from build123d import *

# Parameters (mm, degrees)
SKETCH1_R           = 1.5
SKETCH1_R_2         = 8.5
BOSS_EXTRUDE1_DEPTH = 2
SKETCH2_W           = 35
SKETCH2_H           = 3
BOSS_EXTRUDE2_DEPTH = 117


with BuildPart() as part:
    # Sketch1 → Boss-Extrude1 (new body)
    with BuildSketch(Plane.XY):
        with BuildLine():
            Line((-17.5, 0), (-17.5, -20))
            Line((-17.5, -20), (17.5, -20))
            Line((17.5, -20), (17.5, 0))
            ThreePointArc((17.5, 0), (0, 17.5), (-17.5, 0))
        make_face()
        with Locations((0, 14)):
            Circle(SKETCH1_R, mode=Mode.SUBTRACT)
        with Locations((14, 0)):
            Circle(SKETCH1_R, mode=Mode.SUBTRACT)
        with Locations((0, -14)):
            Circle(SKETCH1_R, mode=Mode.SUBTRACT)
        with Locations((-14, 0)):
            Circle(SKETCH1_R, mode=Mode.SUBTRACT)
        Circle(SKETCH1_R_2, mode=Mode.SUBTRACT)
    extrude(amount=BOSS_EXTRUDE1_DEPTH)

    # Sketch2 → Boss-Extrude2 (add)
    with BuildSketch(Plane(origin=(0, 0, 0), x_dir=(-1, 0, 0), z_dir=(0, 0, -1))):
        with Locations((0, -18.5)):
            Rectangle(SKETCH2_W, SKETCH2_H)
    extrude(amount=BOSS_EXTRUDE2_DEPTH)


solid = part.part
Input: part model. Units: mm. Frame: model coordinates. A direction names the side the tool comes from. Round coordinates to 2 decimals unless told otherwise and drop trailing zeros. Write each loop counter-clockwise with the first axis right and the second up, starting at its lowest first coordinate (ties: lowest second). Pieces come first, ordered by that corner, then holes.
1) Cut plane A-A (x = 0). Return the cut outline in (y, z), then the cut area to 3 significant figures.
2) Cut plane D-D (z = -19). Return the cut outline in (x, y), then the cut area to 3 significant figures.
3) Cut plane B-B (y = -14). Return the cut outline in (x, z).
4) Contact query for flat-ended pins moving along their axis: P1, Ø1, axis at x = 9, z = -29, coming from the +Y side; P2, Ø12, axis at y = -6, z = -60.5, coming from the +X side; P3, Ø5, axis at x = 0, y = -14, coming from the +Z side; P4, Ø5, axis at x = 0, y = 14, coming from the -Z side. Output: stop coordinate, or through.
5) Reachability of faces 5 (the flat face through (0, -17, -58)), 6 (the flat face through (0, -20, -57)) from +Z, -Z, +X, -X, +Y, -Y: full face, straight path, thin tool, end or side. Return the list, or none.
6) Cut plane C-C (x = 14). Return the cut outline in (y, z), then the cut area to 3 significant figures.
7) Draft query along X for faces 1 (the flat face through (-8, -3.3, 0)), 2 (the cylindrical face through (-0.325, 12.536, 0.986)), 3 (the flat face through (17.5, -17.5, -48.4)), 4 (the flat face through (-17.5, -17.5, -48.4)). Return one class per face: pulls with the +X half, pulls with the -X half, needs draft (parallel to the pull), parting line crosses it, or undercut.
8) Ray query, L1, parallel to Y at x = 0, z = 0.95; L2, parallel to Y at x = -6.5, z = -93; L3, parallel to Z at x = -7, y = 15.5. Return the intervals inside material, ascending.
Geometry says:
1. outline: (-20, -117) - (-17, -117) - (-17, 0) - (-15.5, 0) - (-15.5, 2) - (-20, 2) - close; (-12.5, 0) - (-8.5, 0) - (-8.5, 2) - (-12.5, 2) - close; (8.5, 0) - (12.5, 0) - (12.5, 2) - (8.5, 2) - close; (15.5, 0) - (17.5, 0) - (17.5, 2) - (15.5, 2) - close
1. area: 380 mm2
2. outline: (-17.5, -20) - (17.5, -20) - (17.5, -17) - (-17.5, -17) - close
2. area: 105 mm2
3. outline: (-17.5, 0) - (-1.5, 0) - (-1.5, 2) - (-17.5, 2) - close; (1.5, 0) - (17.5, 0) - (17.5, 2) - (1.5, 2) - close
4. P1: stops at y = -17
4. P2: passes through
4. P3: stops at z = 2
4. P4: stops at z = 0
5. face 5: -Z, +X, -X, +Y
5. face 6: +Z, -Z, +X, -X, -Y
6. outline: (-20, -117) - (-17, -117) - (-17, 0) - (-1.5, 0) - (-1.5, 2) - (-20, 2) - close; (1.5, 0) - (10.5, 0) - (10.5, 2) - (1.5, 2) - close
6. area: 406 mm2
7. face 1: needs draft
7. face 2: undercut
7. face 3: pulls with the +X half
7. face 4: pulls with the -X half
8. L1: y = -20 to -15.5, -12.5 to -8.5, 8.5 to 12.5, 15.5 to 17.5
8. L2: y = -20 to -17
8. L3: z = 0 to 2
